Answer from the drawing. Dimensions are ordinates in mm from the lowest x, y and z of the part. Round coordinates to 2 decimals unless told otherwise and drop trailing zeros. Write each loop counter-clockwise with the first axis right and the second up, starting at its lowest first coordinate (ties: lowest second). Pieces come first, ordered by that corner, then holes. Notation, with made-up numbers: (87.25, 76.25) - (138.25, 76.25) arc R23 ccw to (138.25, 115.25) - close; hole circle Ø10 at (17, 36). An arc over 180 degrees is marked (long way). Answer as a JSON object with one key per item and string values.
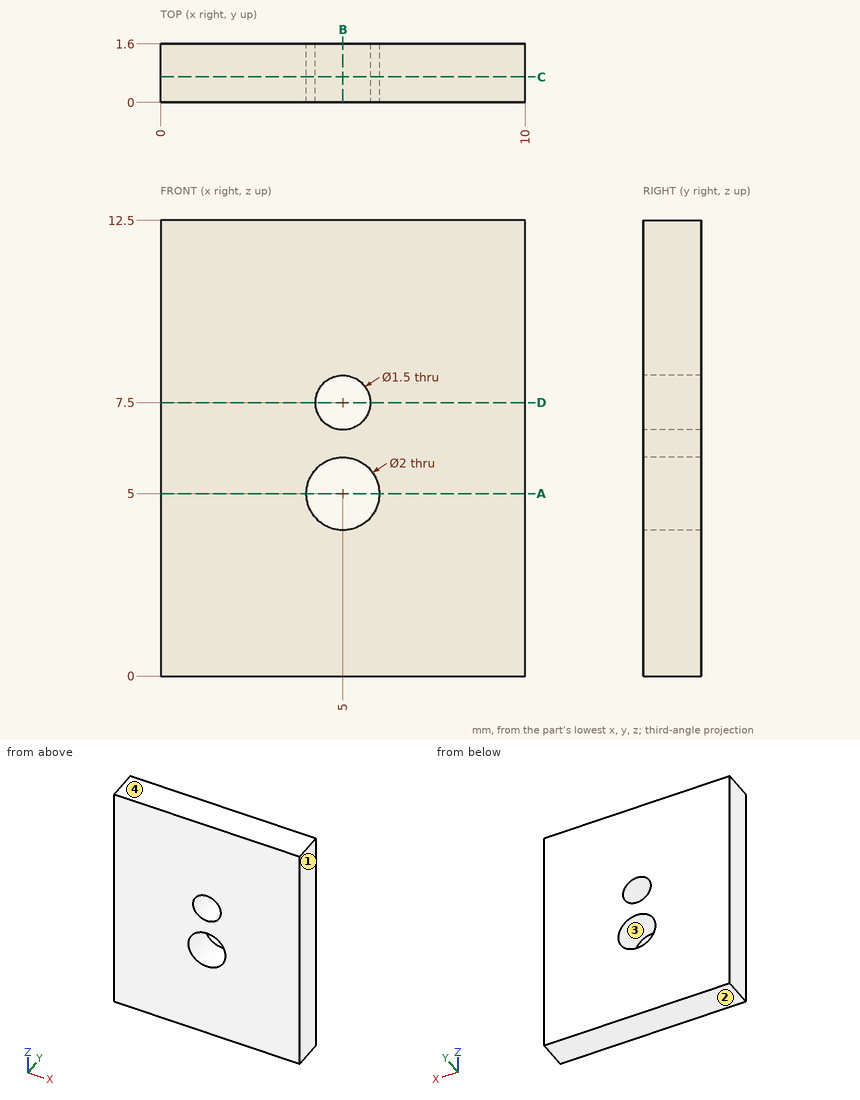
Item 1: A cutting plane is placed at C-C (y = 0.7). Write down the section's boundary in (x, z).
Results found:
{"outline": "(0, 0) - (10, 0) - (10, 12.5) - (0, 12.5) - close; hole circle Ø2 at (5, 5); hole circle Ø1.5 at (5, 7.5)"}
Item 2: A cutting plane is placed at A-A (z = 5). Write down the section's boundary in (x, y).
Results found:
{"outline": "(0, 0) - (4, 0) - (4, 1.6) - (0, 1.6) - close; (6, 0) - (10, 0) - (10, 1.6) - (6, 1.6) - close"}
Item 3: This flat-tipped pin is pushed along its axis until it touches: P1, Ø1.8, axis at x = 5, z = 5, coming from the +Y side. Where does it stop, or does it pass through?
Results found:
{"P1": "through"}
Item 4: Determine the mould class of the marked faces 1, 2, 3 and 4 for opening direction Z: pulls with the +Z half, pulls with the -Z half, needs draft (parallel to the pull), parting line crosses it, or undercut.
Results found:
{"face 1": "needs draft", "face 2": "pulls with the -Z half", "face 3": "undercut", "face 4": "pulls with the +Z half"}
Item 5: A cutting plane is placed at D-D (z = 7.5). Write down the section's boundary in (x, y), and give its area (3 significant figures).
Results found:
{"outline": "(0, 0) - (4.25, 0) - (4.25, 1.6) - (0, 1.6) - close; (5.75, 0) - (10, 0) - (10, 1.6) - (5.75, 1.6) - close", "area": "13.6 mm²"}
Item 6: Consider line 1 along Z through (x, y) = (5, 0.5); line 2 along X through (y, z) = (0.6, 7.75). Determine where each line is inside the solid, lowest interval first.
Results found:
{"line 1": "0 to 4, 6 to 6.75, 8.25 to 12.5", "line 2": "0 to 4.29, 5.71 to 10"}
Item 7: A cutting plane is placed at B-B (x = 5). Write down the section's boundary in (y, z), and give its area (3 significant figures).
Results found:
{"outline": "(0, 0) - (1.6, 0) - (1.6, 4) - (0, 4) - close; (0, 6) - (1.6, 6) - (1.6, 6.75) - (0, 6.75) - close; (0, 8.25) - (1.6, 8.25) - (1.6, 12.5) - (0, 12.5) - close", "area": "14.4 mm²"}
